from build123d import *
from OCP.BRepFilletAPI import BRepFilletAPI_MakeChamfer

# Parameters (mm, degrees)
CROQUIS7_R              = 3.175
CROQUIS7_R_2            = 1.585
CHAFL_N2_SIZE           = 1
CHAFL_N2_SIZE2          = 0.577350269
CROQUIS7_3_R            = 3.175
CROQUIS7_3_R_2          = 1.585
SALIENTE_EXTRUIR2_DEPTH = 855
CHAFL_N3_SIZE           = 1
CHAFL_N3_SIZE2          = 0.577350269


with BuildPart() as part:
    # Barrer4: sweep along a path in Croquis6
    with BuildLine(Plane.XY) as barrer4_path:
        Line((0, 0), (0, 100))
        ThreePointArc((0, 100), (3.620568169, 173.605324125), (14.447316639, 246.5))
        ThreePointArc((14.447316639, 246.5), (208.645238435, 390.471063639), (370.979960645, 211.34))
        Line((370.979960645, 211.34), (370.979960645, 86))
    # Croquis7 → Barrer4 (sweep)
    with BuildSketch(Plane(origin=(0, 0, 0), x_dir=(1, 0, 0), z_dir=(0, 1, 0))):
        Circle(CROQUIS7_R)
        Circle(CROQUIS7_R_2, mode=Mode.SUBTRACT)
    sweep(path=barrer4_path.line)

    # Chafl_n2: one chamfer whose edges measure the first distance from different faces: ONE call of the kernel's chamfer builder (chamfer() names one face for all edges)
    chafl_n2_edges_1 = [part.edges().sort_by_distance(p)[0] for p in [
        (372.564960645, 86, 0),
    ]]
    chafl_n2_side_1 = [part.faces().sort_by_distance(p)[0] for p in [
        (372.564960645, 148.67, 0),
    ]]
    chafl_n2_edges_2 = [part.edges().sort_by_distance(p)[0] for p in [
        (-1.585, 0, 0),
    ]]
    chafl_n2_side_2 = [part.faces().sort_by_distance(p)[0] for p in [
        (-1.585, 50, 0),
    ]]
    chafl_n2 = BRepFilletAPI_MakeChamfer(part.part.solid().wrapped)
    for e in chafl_n2_edges_1:
        chafl_n2.Add(CHAFL_N2_SIZE, CHAFL_N2_SIZE2, e.wrapped, chafl_n2_side_1[0].wrapped)  # the first distance lies on this face
    for e in chafl_n2_edges_2:
        chafl_n2.Add(CHAFL_N2_SIZE, CHAFL_N2_SIZE2, e.wrapped, chafl_n2_side_2[0].wrapped)  # the first distance lies on this face
    add(Compound.cast(chafl_n2.Shape()), mode=Mode.REPLACE)


with BuildPart() as body_2:
    # Croquis7_3 → Saliente-Extruir2 (new body)
    with BuildSketch(Plane(origin=(0, 0, 0), x_dir=(1, 0, 0), z_dir=(0, 1, 0))):
        with Locations(Location((0, 0, 0), (0, 0, 90))):
            Circle(CROQUIS7_3_R)
        with Locations(Location((0, 0, 0), (0, 0, 90))):
            Circle(CROQUIS7_3_R_2, mode=Mode.SUBTRACT)
    extrude(amount=SALIENTE_EXTRUIR2_DEPTH)

    # Chafl_n3
    chafl_n3_edges = [body_2.edges().sort_by_distance(p)[0] for p in [
        (0, 0, 1.585),
        (0, 855, 1.585),
    ]]
    chafl_n3_side = [body_2.faces().sort_by_distance(p)[0] for p in [
        (0, 427.5, 1.585),
    ]]
    chamfer(chafl_n3_edges, length=CHAFL_N3_SIZE, length2=CHAFL_N3_SIZE2, reference=chafl_n3_side[0])


solid = body_2.part
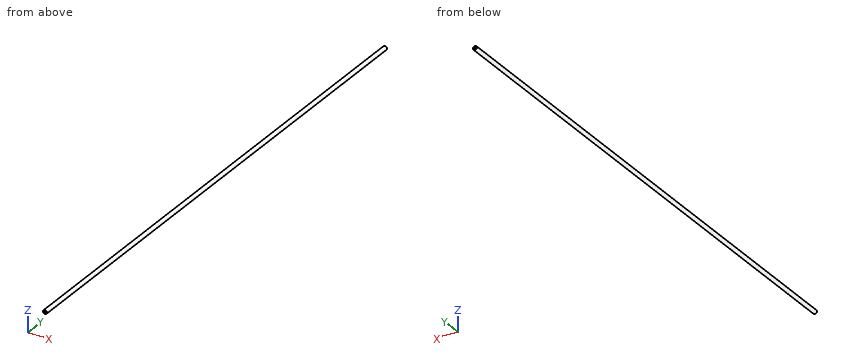
Here's how the part is built. I have some questions about the finished solid (model axes, mm). Coordinates: 2 decimals unless noted, no trailing zeros. Order: outer loops, then holes, each group sorted by start corner. A loop starts at its lowest first (then second) coordinate and runs counter-clockwise, first axis right, second up. Notation, with made-up numbers: M -20,86 L 33,86 A21 ccw 33,118 Z; hole C 23,50.5 d7. An arc over 180 degrees is marked long. Answer as CSV lines item,"result".
Item 1: Imagine slicing it at B-B on z = 0. Write out the boundary of the cut face in (x, y) (3 decimals).
Results found:
outline,"M -3.175,0 L -2.162,0 L -1.585,1 L -1.585,854 L -2.162,855 L -3.175,855 Z; M 1.585,1 L 2.162,0 L 3.175,0 L 3.175,855 L 2.162,855 L 1.585,854 Z"
Item 2: Imagine slicing it at C-C on y = 433.5. Write out the boundary of the cut face in (x, z) (3 decimals).
Results found:
outline,"C 0,0 d6.35; hole C 0,0 d3.17"
Item 3: If I drill on line 1 (X direction, y = 76, z = -0.25); line 2 (X direction, y = 431, z = -0.5); line 3 (X direction, y = 595, z = -2.25), over which ranges is the centre line in solid material (lowest first)?
Results found:
line 1,"-3.17 to -1.57, 1.57 to 3.17"
line 2,"-3.14 to -1.5, 1.5 to 3.14"
line 3,"-2.24 to 2.24"
Item 4: Imagine slicing it at A-A on x = 0. Write out the boundary of the cut face in (y, z) (3 decimals).
Results found:
outline,"M 0,-3.175 L 855,-3.175 L 855,-2.162 L 854,-1.585 L 1,-1.585 L 0,-2.162 Z; M 0,2.162 L 1,1.585 L 854,1.585 L 855,2.162 L 855,3.175 L 0,3.175 Z"
